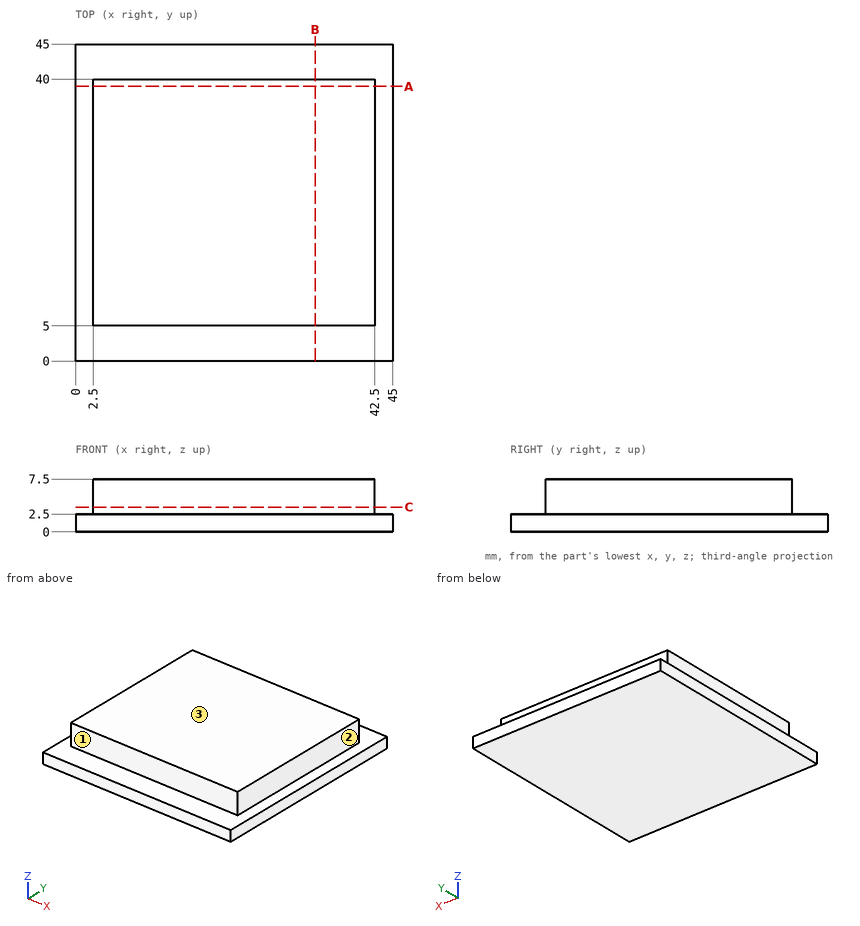
Study the drawing (mm; zero at the part's minimum x, y, z) and answer. A direction names the side the tool comes from. Coordinates: 2 decimals unless noted, no trailing zeros. Loops run counter-clockwise (first coordinate to the right, second up) from the corner with the lowest first, then second, coordinate; pieces in that order, holes last. Notation, with made-up numbers: M 18.5,30.5 L 28.5,30.5 A12 cw 28.5,47.5 Z; hole C 88.25,61 d2. An arc over 180 degrees is marked long. Answer in a Markdown table with one row per item.
1) Find the intervals of material crossed by probe 1 along X at (y, z) = (31, 3.5); probe 2 along Y at (x, z) = (26, 3.5); probe 3 along Z at (x, y) = (26, 3), in increasing order.
Answers below:
| item | result |
|---|---|
| probe 1 | 2.5 to 42.5 |
| probe 2 | 5 to 40 |
| probe 3 | 0 to 2.5 |
2) Find section B-B (x = 34). Determine the outline of the cut face in (y, z).
Answers below:
| item | result |
|---|---|
| outline | M 0,0 L 45,0 L 45,2.5 L 40,2.5 L 40,7.5 L 5,7.5 L 5,2.5 L 0,2.5 Z |
3) Find section C-C (z = 3.5). Determine the outline of the cut face in (x, y).
Answers below:
| item | result |
|---|---|
| outline | M 2.5,5 L 42.5,5 L 42.5,40 L 2.5,40 Z |
4) Which of the six approach directions +Z, -Z, +X, -X, +Y, -Y give full straight-line access (tool end or side, diameter ignored) to the marked faces 1, 2 and 3?
Answers below:
| item | result |
|---|---|
| face 1 | +Z, +X, -X, -Y |
| face 2 | +Z, +X, +Y, -Y |
| face 3 | +Z, +X, -X, +Y, -Y |
5) Find section A-A (y = 39). Determine the outline of the cut face in (x, z), then the cut area to 4 significant figures.
Answers below:
| item | result |
|---|---|
| outline | M 0,0 L 45,0 L 45,2.5 L 42.5,2.5 L 42.5,7.5 L 2.5,7.5 L 2.5,2.5 L 0,2.5 Z |
| area | 312.5 mm^2 |
6) Given pin 1 (1 mm diameter, centred on x = 40, y = 8.5, fed in from -Z); pin 2 (2.5 mm diameter, centred on x = 23.5, z = 4, fed in from -Y), each flat-ended and moving along its own axis, determine where each tip first touches the part or whether it passes through.
Answers below:
| item | result |
|---|---|
| pin 1 | z = 0 |
| pin 2 | y = 5 |
